Can you work these out from the drawing? Everything is in mm from the part's minimum corner. Round coordinates to 2 decimals unless told otherwise and drop trailing zeros. Order: outer loops, then holes, each group sorted by start corner. A loop starts at its lowest first (then second) coordinate and runs counter-clockwise, first axis right, second up. Notation, with made-up numbers: (-8, 29) -> (9, 29) arc R13 ccw to (9, 38) -> close; hole circle Ø5 at (59, 58). An arc over 180 degrees is marked (long way). One line per item, written item: value.
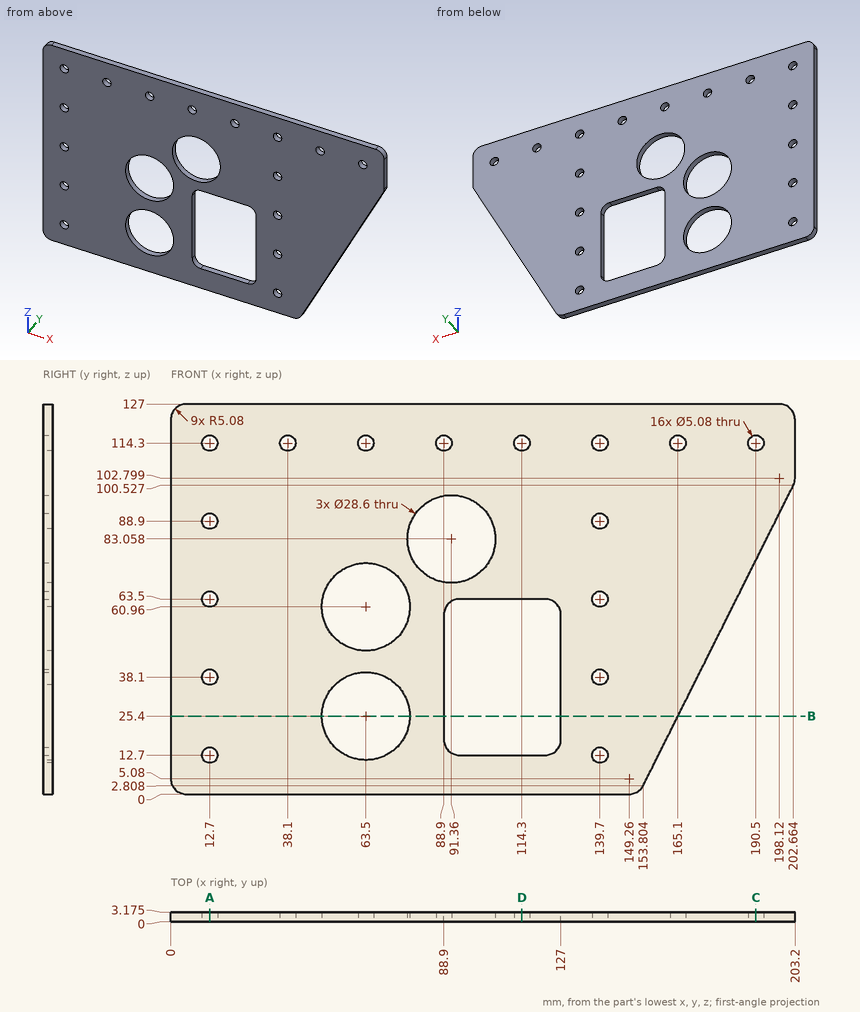
Q1. Will these pins go through, and if not, where does the flat tip stop? pin 1 Ø3 at (x, z) = (12.7, 114.3) entering from +Y; pin 2 Ø12 at (x, z) = (57.5, 70.5) entering from +Y (3 decimals).
Answers below:
pin 1: through
pin 2: y = 3.175
Q2. I want a section at C-C on x = 190.5. List the corners of the cut face in (y, z) for me (1 decimal), plus the area to 3 significant figures.
Answers below:
outline: (0, 76.2) -> (3.2, 76.2) -> (3.2, 111.8) -> (0, 111.8) -> close; (0, 116.8) -> (3.2, 116.8) -> (3.2, 127) -> (0, 127) -> close
area: 145 mm^2
Q3. Please list where these lines run through material, in increasing order: line 1 along Z through (x, y) = (139.7, 0.85); line 2 along X through (y, z) = (0.6, 56.5); line 3 along X through (y, z) = (1.3, 56).
Answers below:
line 1: 0 to 10.16, 15.24 to 35.56, 40.64 to 60.96, 66.04 to 86.36, 91.44 to 111.76, 116.84 to 127
line 2: 0 to 49.91, 77.09 to 88.9, 127 to 180.65
line 3: 0 to 50.09, 76.91 to 88.9, 127 to 180.4
Q4. I want a section at B-B on z = 25.4. List the corners of the cut face in (x, y) for me (1 decimal).
Answers below:
outline: (0, 0) -> (49.2, 0) -> (49.2, 3.2) -> (0, 3.2) -> close; (77.8, 0) -> (88.9, 0) -> (88.9, 3.2) -> (77.8, 3.2) -> close; (127, 0) -> (165.1, 0) -> (165.1, 3.2) -> (127, 3.2) -> close
Q5. I want a section at D-D on x = 114.3. List the corners of the cut face in (y, z) for me (1 decimal), plus the area to 3 significant figures.
Answers below:
outline: (0, 0) -> (3.2, 0) -> (3.2, 12.7) -> (0, 12.7) -> close; (0, 63.5) -> (3.2, 63.5) -> (3.2, 111.8) -> (0, 111.8) -> close; (0, 116.8) -> (3.2, 116.8) -> (3.2, 127) -> (0, 127) -> close
area: 226 mm^2
Q6. I want a section at A-A on x = 12.7. List the corners of the cut face in (y, z) for me (1 decimal).
Answers below:
outline: (0, 0) -> (3.2, 0) -> (3.2, 10.2) -> (0, 10.2) -> close; (0, 15.2) -> (3.2, 15.2) -> (3.2, 35.6) -> (0, 35.6) -> close; (0, 40.6) -> (3.2, 40.6) -> (3.2, 61) -> (0, 61) -> close; (0, 66) -> (3.2, 66) -> (3.2, 86.4) -> (0, 86.4) -> close; (0, 91.4) -> (3.2, 91.4) -> (3.2, 111.8) -> (0, 111.8) -> close; (0, 116.8) -> (3.2, 116.8) -> (3.2, 127) -> (0, 127) -> close
